```python
from build123d import *

# Parameters (mm, degrees)
F1_DEPTH = 76.2
F2_R     = 1.9685
F3_DEPTH = 2.033


with BuildPart() as f1:
    # F0 (on Front) → F1 (new body, symmetric)
    with BuildSketch(Plane.XZ):
        Polygon((0, 0), (0, 25.4), (-2.032, 25.4), (-2.032, 2.032), (-5.588, 2.032), (-5.588, 8.89), (-7.62, 8.89), (-7.62, 0), align=None)
    extrude(amount=F1_DEPTH, both=True)

    # F2 (on face) → F3 (cut, through all)
    with BuildSketch(Plane(origin=(-2.032, 0, 0), x_dir=(0, -1, 0), z_dir=(-1, 0, 0))):
        with Locations((-60.325, 18.7325)):
            Circle(F2_R)
        with Locations((0, 18.7325)):
            Circle(F2_R)
        with Locations((60.325, 18.7325)):
            Circle(F2_R)
    extrude(amount=-F3_DEPTH, mode=Mode.SUBTRACT)


solid = f1.part
```
CAD build for the part. Positions are in the model's coordinates, mm. A direction names the side the tool comes from. Give positions to 0.01 mm unless a question says otherwise; leave off trailing zeros. Order: outer loops, then holes, each group sorted by start corner. A loop starts at its lowest first (then second) coordinate and runs counter-clockwise, first axis right, second up.
(1) Saw through at D-D, the plane x = -4. Give the cut face in (y, z), then the cut area to 3 significant figures.
(2) Drill centre lines: L1, parallel to X at y = 56.5, z = 7; L2, parallel to Z at x = -0.8, y = 0; L3, parallel to Z at x = -4, y = -62. Where is each one in solid material? Low to high.
(3) Mould opens along Z. For faces 1 (the flat face through (-2.032, -1, 14)), 2 (the flat face through (-4, -1, 0)), 3 (the cylindrical face through (-1.03, -58.36, 18.82)) say: released by +Z, released by -Z, zero draft, split by the parting line, or undercut.
(4) Flat gauge pins, fed straight in: pin 1 (6.5 mm diameter, centred on y = 0, z = 18.73, fed in from -X); pin 2 (1.1 mm diameter, centred on x = -4, y = -15, fed in from +Z); pin 3 (1 mm diameter, centred on x = -6, y = -1, fed in from +Z). Where does each tip first touch, or does it go through?
(5) Saw through at B-B, the plane y = 0. Give the cut face in (x, z), then the cut area to 3 significant figures.
(6) Saw through at A-A, the plane z = 6.25. Give the cut face in (x, y), then the cut area to 3 significant figures.
(7) Saw through at C-C, the plane y = 44. Give the cut face in (x, z).
(8) Tool access for faces 4 (the flat face through (-5.588, -1, 5)), 5 (the cylindrical face through (-1.03, 0.256, 20.684)): list every direction of +Z, -Z, +X, -X, +Y, -Y with a clear straight run to the whole face (end or side of a thin tool).
Results found:
1. outline: (-76.2, 0) - (76.2, 0) - (76.2, 2.03) - (-76.2, 2.03) - close
1. area: 310 mm2
2. L1: x = -7.62 to -5.59, -2.03 to 0
2. L2: z = 0 to 16.76, 20.7 to 25.4
2. L3: z = 0 to 2.03
3. face 1: zero draft
3. face 2: released by -Z
3. face 3: undercut
4. pin 1: stops at x = -2.03
4. pin 2: stops at z = 2.03
4. pin 3: stops at z = 8.89
5. outline: (-7.62, 0) - (0, 0) - (0, 16.76) - (-2.03, 16.76) - (-2.03, 2.03) - (-5.59, 2.03) - (-5.59, 8.89) - (-7.62, 8.89) - close; (-2.03, 20.7) - (0, 20.7) - (0, 25.4) - (-2.03, 25.4) - close
5. area: 68.9 mm2
6. outline: (-7.62, -76.2) - (-5.59, -76.2) - (-5.59, 76.2) - (-7.62, 76.2) - close; (-2.03, -76.2) - (0, -76.2) - (0, 76.2) - (-2.03, 76.2) - close
6. area: 619 mm2
7. outline: (-7.62, 0) - (0, 0) - (0, 25.4) - (-2.03, 25.4) - (-2.03, 2.03) - (-5.59, 2.03) - (-5.59, 8.89) - (-7.62, 8.89) - close
8. face 4: +Z, +Y, -Y
8. face 5: +X, -X
